Check sheet for the modelled part. Datum: model origin and axes. Units: mm. Face numbers are marked on the shaded views. A direction names the side the tool comes from. Round coordinates to 2 decimals unless told otherwise and drop trailing zeros. Order: outer loops, then holes, each group sorted by start corner. A loop starts at its lowest first (then second) coordinate and runs counter-clockwise, first axis right, second up.
(1) Mould release check, pull along X, two halves, no side actions. Record for the marked faces 1 and 2: released by +X, released by -X, zero draft, split by the parting line, or undercut.
(2) Tool access check on the marked faces 3 and 4. Record the directions out of +Z, -Z, +X, -X, +Y, -Y that give a thin tool (end or side, any length) a straight path to the whole face; none if there is none.
(3) Thickness scan on probe 1 along Y at (x, z) = (8, 2.75); probe 2 along Z at (x, y) = (-0.25, 11); probe 3 along X at (y, z) = (17.5, -8). Record the ranges inside material, lowest first.
(4) Depth check by flat-ended pin: pin 1 (1 mm diameter, centred on x = 4.5, z = 2, fed in from +Y); pin 2 (1.5 mm diameter, centred on x = 7, y = 15.5, fed in from +Z); pin 3 (5 mm diameter, centred on x = -7.5, y = 23, fed in from +Z). Enter the tip coordinate at first touch or a pass-through.
(5) Sectioned sample at A-A, the plane y = 8.5. Enter the section's corners in (x, z), and give its area (3 significant figures).
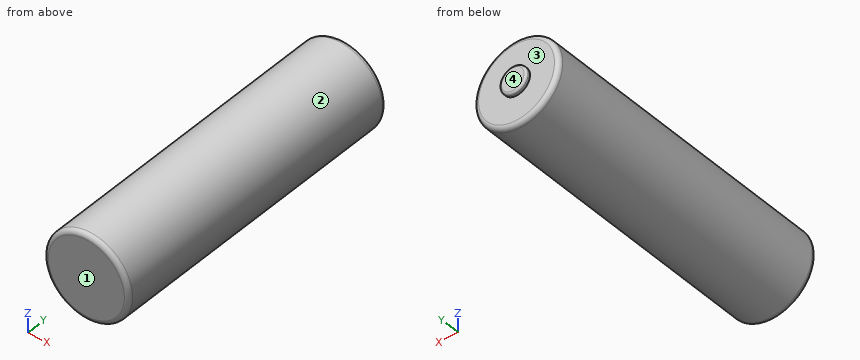
```python
from build123d import *

# Parameters (mm, degrees)
SKETCH1_R                = 9.45
BOSS_EXTRUDE1_DEPTH      = 35
BOSS_EXTRUDE1_DEPTH_BACK = 35
SKETCH2_R                = 9.45
SKETCH2_R_2              = 3
CUT_EXTRUDE1_DEPTH       = 1
FILLET1_R                = 0.5
FILLET2_R                = 1


with BuildPart() as part:
    # Sketch1 → Boss-Extrude1 (new body, two sides)
    with BuildSketch(Plane(origin=(0, 0, 0), x_dir=(1, 0, 0), z_dir=(0, 1, 0))) as boss_extrude1_sk:
        Circle(SKETCH1_R)
    extrude(amount=BOSS_EXTRUDE1_DEPTH)
    extrude(boss_extrude1_sk.sketch, amount=-BOSS_EXTRUDE1_DEPTH_BACK)

    # Sketch2 → Cut-Extrude1 (cut)
    with BuildSketch(Plane(origin=(0, 35, 0), x_dir=(1, 0, 0), z_dir=(0, 1, 0))):
        Circle(SKETCH2_R)
        Circle(SKETCH2_R_2, mode=Mode.SUBTRACT)
    extrude(amount=-CUT_EXTRUDE1_DEPTH, mode=Mode.SUBTRACT)

    # Fillet1
    fillet1_edges = [part.edges().sort_by_distance(p)[0] for p in [
        (-3, 35, 0),
    ]]
    fillet(fillet1_edges, radius=FILLET1_R)

    # Fillet2
    fillet2_edges = [part.edges().sort_by_distance(p)[0] for p in [
        (-9.45, -35, 0),
        (-9.45, 34, 0),
    ]]
    fillet(fillet2_edges, radius=FILLET2_R)


solid = part.part
```
Derived:
1. face 1: zero draft
1. face 2: split by the parting line
2. face 3: +Y
2. face 4: +Z, -Z, +X, -X, +Y
3. probe 1: y = -35 to 34
3. probe 2: z = -9.45 to 9.45
3. probe 3: x = -5.03 to 5.03
4. pin 1: stops at y = 34
4. pin 2: stops at z = 7.09
4. pin 3: stops at z = 8.02
5. outline: circle Ø18.9 at (0, 0)
5. area: 281 mm2
